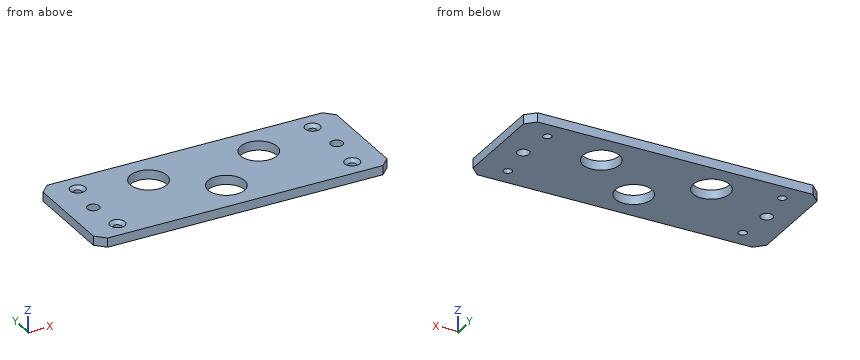
from build123d import *

# Parameters (mm, degrees)
SKETCH1_W                                       = 203.2
SKETCH1_H                                       = 76.2
BOSS_EXTRUDE1_DEPTH                             = 6.35
M8_CLEARANCE_HOLE1_D                            = 8.4
M8_CLEARANCE_HOLE1_DEPTH                        = 10.668
M8_CLEARANCE_HOLE1_TIP                          = 2.5236146
CHAMFER1_SIZE                                   = 6.35
CSK_FOR_M5_FLAT_HEAD_MACHINE_SCREW1_D           = 5.8
CSK_FOR_M5_FLAT_HEAD_MACHINE_SCREW1_CSINK_D     = 10.4
CSK_FOR_M5_FLAT_HEAD_MACHINE_SCREW1_CSINK_ANGLE = 90
F_1_1_DIAMETER_HOLE1_D                          = 25.4


with BuildPart() as part:
    # Sketch1 → Boss-Extrude1 (new body)
    with BuildSketch(Plane.XY):
        Rectangle(SKETCH1_W, SKETCH1_H)
    extrude(amount=BOSS_EXTRUDE1_DEPTH)

    # M8 Clearance Hole1
    with Locations(Plane.XY.offset(6.35)):
        with Locations((84.25, 0), (-84.25, 0)):
            Hole(M8_CLEARANCE_HOLE1_D / 2, depth=M8_CLEARANCE_HOLE1_DEPTH)
            with Locations((0, 0, -(M8_CLEARANCE_HOLE1_DEPTH + M8_CLEARANCE_HOLE1_TIP / 2))):  # 118° drill point
                Cone(0, M8_CLEARANCE_HOLE1_D / 2, M8_CLEARANCE_HOLE1_TIP, mode=Mode.SUBTRACT)

    # Chamfer1
    chamfer1_edges = [part.edges().sort_by_distance(p)[0] for p in [
        (-101.6, 38.1, 3.175),
        (101.6, 38.1, 3.175),
        (101.6, -38.1, 3.175),
        (-101.6, -38.1, 3.175),
    ]]
    chamfer(chamfer1_edges, length=CHAMFER1_SIZE)

    # CSK for M5 Flat Head Machine Screw1 (through all)
    with Locations(Plane.XY.offset(6.35)):
        with Locations((81.25, 25), (81.25, -25), (-81.25, -25), (-81.25, 25)):
            CounterSinkHole(CSK_FOR_M5_FLAT_HEAD_MACHINE_SCREW1_D / 2, CSK_FOR_M5_FLAT_HEAD_MACHINE_SCREW1_CSINK_D / 2, counter_sink_angle=CSK_FOR_M5_FLAT_HEAD_MACHINE_SCREW1_CSINK_ANGLE)

    # 1 (1) Diameter Hole1 (through all)
    with Locations(Plane.XY.offset(6.35)):
        with Locations((0, -14.2875), (-38.1, 14.2875), (38.1, 14.2875)):
            Hole(F_1_1_DIAMETER_HOLE1_D / 2)


solid = part.part
Work out the finished part from the listing and answer in its coordinate system (mm). Coordinates: 2 decimals unless noted, no trailing zeros. Write each loop counter-clockwise with the first axis right and the second up, starting at its lowest first coordinate (ties: lowest second). Pieces come first, ordered by that corner, then holes. Notation, with made-up numbers: M 7.5,47 L 51.5,47 A16 cw 51.5,76 Z; hole C -1.5,70.25 d5. An arc over 180 degrees is marked long. Write item = value, one per line.
1. The part is cut by section C-C (y = 6). Determine the outline of the cut face in (x, z), then the cut area to 3 significant figures.
Solution:
outline = M -101.6,0 L -47.72,0 L -47.72,6.35 L -101.6,6.35 Z; M -28.48,0 L 28.48,0 L 28.48,6.35 L -28.48,6.35 Z; M 47.72,0 L 101.6,0 L 101.6,6.35 L 47.72,6.35 Z
area = 1,050 mm2
2. The part is cut by section D-D (y = -25). Determine the outline of the cut face in (x, z), then the cut area to 3 significant figures.
Solution:
outline = M -101.6,0 L -84.15,0 L -84.15,4.05 L -86.45,6.35 L -101.6,6.35 Z; M -78.35,0 L -6.82,0 L -6.82,6.35 L -76.05,6.35 L -78.35,4.05 Z; M 6.82,0 L 78.35,0 L 78.35,4.05 L 76.05,6.35 L 6.82,6.35 Z; M 84.15,0 L 101.6,0 L 101.6,6.35 L 86.45,6.35 L 84.15,4.05 Z
area = 1,120 mm2
3. The part is cut by section A-A (x = -36.5). Determine the outline of the cut face in (y, z), then the cut area to 3 significant figures.
Solution:
outline = M -38.1,0 L 1.69,0 L 1.69,6.35 L -38.1,6.35 Z; M 26.89,0 L 38.1,0 L 38.1,6.35 L 26.89,6.35 Z
area = 324 mm2
4. Straight lines are drawn through the part: line 1 (X direction, y = -0.5, z = 0.75); line 2 (Y direction, x = -81.5, z = 3.25); line 3 (X direction, y = 25, z = 3.05). For each, find the intervals that lie inside material, in ascending order. Write a range as from..to.
Solution:
line_1 = -101.6..-88.42, -80.08..80.08, 88.42..101.6
line_2 = -38.1..-27.89, -22.11..-3.17, 3.17..22.11, 27.89..38.1
line_3 = -101.6..-84.15, -78.35..-44.92, -31.28..31.28, 44.92..78.35, 84.15..101.6
5. Flat-ended cylindrical pins translate along their axes: pin 1 (15 mm diameter, centred on x = 0, y = -14.29, fed in from +Z) (1 decimal); pin 2 (6.5 mm diameter, centred on x = 81.25, y = -25, fed in from +Z). Find the tip coordinate at first contact, or state that the pin passes through.
Solution:
pin_1 = through
pin_2 = 4.4
6. The part is cut by section B-B (y = 25). Determine the outline of the cut face in (x, z), then the cut area to 3 significant figures.
Solution:
outline = M -101.6,0 L -84.15,0 L -84.15,4.05 L -86.45,6.35 L -101.6,6.35 Z; M -78.35,0 L -44.92,0 L -44.92,6.35 L -76.05,6.35 L -78.35,4.05 Z; M -31.28,0 L 31.28,0 L 31.28,6.35 L -31.28,6.35 Z; M 44.92,0 L 78.35,0 L 78.35,4.05 L 76.05,6.35 L 44.92,6.35 Z; M 84.15,0 L 101.6,0 L 101.6,6.35 L 86.45,6.35 L 84.15,4.05 Z
area = 1,030 mm2
